The listing builds one solid part. Answer for the finished solid, in the listing's coordinates (mm). A direction names the side the tool comes from. Give positions to 0.01 mm unless a question says otherwise; leave off trailing zeros. Write each loop counter-clockwise with the first axis right and the second up, starting at its lowest first coordinate (ties: lowest second). Pieces come first, ordered by that corner, then holes. Notation, with made-up numbers: M 86,48 L 126,48 A21 cw 126,58 Z; hole C -6,46 d7. An arc over 180 degrees is marked long. Answer as a JSON object with one key per item and string values.
Solid Edge part; units mm, degrees
sketch "Sketch1" plane through (0, 0, 0) normal (0, -1, 0) x (1, 0, 0)
  line L0 (65.1, -3) -> (0, -3)
  line L1 (0, 0) -> (0, -3)
  line L2 (65.1, 0) -> (0, 0)
  line L3 (65.1, 0) -> (65.1, -3)
  line L4 (61.2, 8.9375) -> (61.2, 6.675)
  line L5 (61.2, 6.675) -> (45.2, 6.675)
  line L6 (45.2, 6.675) -> (45.2, 2.4125)
  line L7 (45.2, 2.4125) -> (53.2, 2.4125)
  line L8 (53.2, 2.4125) -> (53.2, 0)
  line L9 (54.2, 0) -> (53.2, 0)
  line L10 (54.2, 3.4125) -> (54.2, 0)
  line L11 (46.2, 3.4125) -> (54.2, 3.4125)
  line L12 (46.2, 5.675) -> (46.2, 3.4125)
  line L13 (62.2, 5.675) -> (46.2, 5.675)
  line L14 (62.2, 9.9375) -> (62.2, 5.675)
  line L15 (54.2, 9.9375) -> (62.2, 9.9375)
  line L16 (54.2, 12.35) -> (54.2, 9.9375)
  line L17 (54.2, 12.35) -> (53.2, 12.35)
  line L18 (53.2, 12.35) -> (53.2, 8.9375)
  line L19 (53.2, 8.9375) -> (61.2, 8.9375)
  line L20 (65.1, 15.35) -> (42.3, 15.35)
  line L21 (42.3, 15.35) -> (42.3, 12.35)
  line L22 (42.3, 12.35) -> (65.1, 12.35)
  line L23 (65.1, 12.35) -> (65.1, 15.35)
  line L24 (65.1, 34.95) -> (42.3, 34.95)
  line L25 (42.3, 34.95) -> (42.3, 37.95)
  line L26 (42.3, 37.95) -> (65.1, 37.95)
  line L27 (65.1, 37.95) -> (65.1, 34.95)
  line L28 (54.2, 37.95) -> (54.2, 40.3625)
  line L29 (54.2, 40.3625) -> (62.2, 40.3625)
  line L30 (62.2, 40.3625) -> (62.2, 44.625)
  line L31 (62.2, 44.625) -> (46.2, 44.625)
  line L32 (46.2, 44.625) -> (46.2, 46.8875)
  line L33 (46.2, 46.8875) -> (54.2, 46.8875)
  line L34 (54.2, 46.8875) -> (54.2, 50.3)
  line L35 (54.2, 50.3) -> (53.2, 50.3)
  line L36 (53.2, 47.8875) -> (53.2, 50.3)
  line L37 (45.2, 47.8875) -> (53.2, 47.8875)
  line L38 (45.2, 43.625) -> (45.2, 47.8875)
  line L39 (61.2, 43.625) -> (45.2, 43.625)
  line L40 (61.2, 41.3625) -> (61.2, 43.625)
  line L41 (53.2, 41.3625) -> (61.2, 41.3625)
  line L42 (53.2, 37.95) -> (53.2, 41.3625)
  line L43 (54.2, 37.95) -> (53.2, 37.95)
  line L44 (65.1, 50.3) -> (0, 50.3)
  line L45 (0, 50.3) -> (0, 53.3)
  line L46 (65.1, 53.3) -> (0, 53.3)
  line L47 (65.1, 50.3) -> (65.1, 53.3)
extrude "Protrusion1" add sketch "Sketch1" along normal blind 6
sketch "Sketch2" plane through (65.1, -3, 13.15) normal (1, 0, 0) x (0, 0, -1)
  line L0 (-2.2, -1) -> (-2.2, 1)
  line L1 (-0.6, 1) -> (-2.2, 1)
  line L2 (-0.6, -1) -> (-0.6, 1)
  line L3 (-2.2, -1) -> (-0.6, -1)
  line L4 (-21.8, -1) -> (-23.4, -1)
  line L5 (-23.4, -1) -> (-23.4, 1)
  line L6 (-23.4, 1) -> (-21.8, 1)
  line L7 (-21.8, -1) -> (-21.8, 1)
extrude "Cutout1" cut sketch "Sketch2" against normal up to next
sketch "Sketch3" plane through (0, -3, 51.8) normal (-1, 0, 0) x (0, 0, -1)
  line L0 (-7.6, 6) -> (-7.6, 0)
  arc A0 (-4.4, 0) -> (-7.6, 0) centre (-6, 0) cw
  line L1 (-4.4, 0) -> (-4.4, 6)
  arc A1 (-7.6, 6) -> (-4.4, 6) centre (-6, 6) cw
  line L2 (-1.5, -3) -> (-1.5, 9)
  line L3 (-1.5, 9) -> (-10.5, 9)
  line L4 (-10.5, 9) -> (-10.5, -3)
  line L5 (-10.5, -3) -> (-1.5, -3)
  line L6 (54.8, -3) -> (54.8, 9)
  line L7 (54.8, 9) -> (63.8, 9)
  line L8 (63.8, 9) -> (63.8, -3)
  line L9 (63.8, -3) -> (54.8, -3)
  arc A2 (60.9, 6) -> (57.7, 6) centre (59.3, 6) ccw
  line L10 (57.7, 0) -> (57.7, 6)
  arc A3 (57.7, 0) -> (60.9, 0) centre (59.3, 0) ccw
  line L11 (60.9, 6) -> (60.9, 0)
extrude "ProtrusiónExtruida_4" add sketch "Sketch3" against normal blind 3
fillet "Redondeo_2" radius 3 6 edges at (1.5, -12, -3) (1.5, -12, -12) (1.5, 0, -12) (1.5, -12, 53.3) (1.5, -12, 62.3) (1.5, 0, 62.3)
sketch "Sketch4" plane through (65.1, -3, 13.85) normal (1, 0, 0) x (0, -1, 0)
  line L0 (7, 1.5) -> (7, -24.1)
  line L1 (7, -24.1) -> (3, -24.1)
  line L2 (3, -24.1) -> (3, 1.5)
  line L3 (3, 1.5) -> (7, 1.5)
extrude "ProtrusiónExtruida_5" add sketch "Sketch4" against normal blind 22.8
sketch "Sketch5" plane through (53.7, -10, 25.15) normal (0, -1, 0) x (0, 0, -1)
  circle A0 centre (0, 0) radius 4.725
extrude "VaciadoExtruido_7" cut sketch "Sketch5" against normal blind 3
fillet "Redondeo_3" [suppressed]
1. Consider line 1 along X through (y, z) = (-8.3, 25.15) (3 decimals); line 2 along Z through (x, y) = (19.5, -5.25); line 3 along Y through (x, z) = (47, 30.5). Determine where each line is inside the solid, lowest interval first.
Verdict:
{"line 1": "x = 42.3 to 48.975, 58.425 to 65.1", "line 2": "z = -3 to 0, 50.3 to 53.3", "line 3": "y = -10 to -6"}
2. A cutting plane is placed at B-B, the plane z = -7.5. Give the vertices of the cut face in (x, y).
Verdict:
{"outline": "M 0,-12 L 3,-12 L 3,-10.6 L 0,-10.6 Z; M 0,-1.4 L 3,-1.4 L 3,0 L 0,0 Z"}
3. For faces 1 (the flat face through (50, -3, 3.412)), 2 (the flat face through (3, -6, 56)), 3 (the cylindrical face through (1.5, -10.6, 57.8)), 4 (the flat face through (54, -6, 25)), determine the directions among +Z, -Z, +X, -X, +Y, -Y from which every point of the face is accessible in a straight line to the end or side of a thin tool.
Verdict:
{"face 1": "+X, +Y, -Y", "face 2": "+Z, +X, +Y, -Y", "face 3": "+X, -X", "face 4": "+X, -X, +Y"}
4. Flat-ended cylindrical pins translate along their axes: pin 1 (5 mm diameter, centred on x = 53.5, y = -3.5, fed in from +Z); pin 2 (0.6 mm diameter, centred on x = 52, y = -3, fed in from -Z); pin 3 (1 mm diameter, centred on y = -5.5, z = -3, fed in from -X); pin 4 (0.7 mm diameter, centred on y = -3, z = 4.5, fed in from +X). Find the tip coordinate at first contact, or state that the pin passes through.
Verdict:
{"pin 1": "stops at z = 53.3", "pin 2": "stops at z = -3", "pin 3": "stops at x = 0", "pin 4": "stops at x = 46.2"}
5. A cutting plane is placed at C-C, the plane x = 43.5. Give the vertices of the cut face in (y, z), plus the area to 3 significant figures.
Verdict:
{"outline": "M -10,12.35 L 0,12.35 L 0,15.35 L -2,15.35 L -2,13.75 L -4,13.75 L -4,15.35 L -6,15.35 L -6,34.95 L -4,34.95 L -4,36.55 L -2,36.55 L -2,34.95 L 0,34.95 L 0,37.95 L -10,37.95 Z; M -6,-3 L 0,-3 L 0,0 L -6,0 Z; M -6,50.3 L 0,50.3 L 0,53.3 L -6,53.3 Z", "area": "168 mm2"}
6. The mould has two halves that part along Y. Classify faces 5 (the flat face through (1, -7, 53.3)), 6 (the flat face through (1, -6, -5.9)), 7 (the cylindrical face through (1.52, -11.1, 61.44)): released by +Y, released by -Y, zero draft, split by the parting line, or undercut.
Verdict:
{"face 5": "zero draft", "face 6": "undercut", "face 7": "released by -Y"}
7. A cutting plane is placed at A-A, the plane x = 30. Give the vertices of the cut face in (y, z).
Verdict:
{"outline": "M -6,-3 L 0,-3 L 0,0 L -6,0 Z; M -6,50.3 L 0,50.3 L 0,53.3 L -6,53.3 Z"}
8. A cutting plane is placed at D-D, the plane z = 25.15. Give the vertices of the cut face in (x, y) (3 decimals).
Verdict:
{"outline": "M 42.3,-10 L 48.975,-10 L 48.975,-7 L 58.425,-7 L 58.425,-10 L 65.1,-10 L 65.1,-6 L 42.3,-6 Z"}
